```python
from build123d import *

# Parameters (mm, degrees)
SKETCH1_W           = 20
SKETCH1_H           = 20
SKETCH1_R           = 1.25
SKETCH1_R_2         = 2.625
BOSS_EXTRUDE1_DEPTH = 4


with BuildPart() as part:
    # Sketch1 → Boss-Extrude1 (new body)
    with BuildSketch(Plane(origin=(0, 0, 0), x_dir=(1, 0, 0), z_dir=(0, 1, 0))):
        with Locations((10, 10)):
            Rectangle(SKETCH1_W, SKETCH1_H)
        with Locations((17, 17)):
            Circle(SKETCH1_R, mode=Mode.SUBTRACT)
        with Locations((4.4625, 10)):
            Circle(SKETCH1_R_2, mode=Mode.SUBTRACT)
        with Locations((17, 3)):
            Circle(SKETCH1_R, mode=Mode.SUBTRACT)
        with BuildLine():
            Line((13.925, 7), (13.925, 13))
            ThreePointArc((13.925, 13), (15.5, 14.575), (17.075, 13))
            Line((17.075, 13), (17.075, 7))
            ThreePointArc((17.075, 7), (15.5, 5.425), (13.925, 7))
        make_face(mode=Mode.SUBTRACT)
        with BuildLine():
            Line((8.925, 7), (8.925, 13))
            ThreePointArc((8.925, 13), (10.5, 14.575), (12.075, 13))
            Line((12.075, 13), (12.075, 7))
            ThreePointArc((12.075, 7), (10.5, 5.425), (8.925, 7))
        make_face(mode=Mode.SUBTRACT)
    extrude(amount=-BOSS_EXTRUDE1_DEPTH)


solid = part.part
```
The listing builds one solid part. Answer for the finished solid, in the listing's coordinates (mm). A direction names the side the tool comes from. Give positions to 0.01 mm unless a question says otherwise; leave off trailing zeros. Order: outer loops, then holes, each group sorted by start corner. A loop starts at its lowest first (then second) coordinate and runs counter-clockwise, first axis right, second up.
1) Determine the mould class of faces 1 (the face through (10, -2, 0)), 2 (the face through (10.465, -1.972, -14.575)), 3 (the face through (8, -4, -10)) for opening direction Z: pulls with the +Z half, pulls with the -Z half, needs draft (parallel to the pull), parting line crosses it, or undercut.
Reported:
face 1: pulls with the +Z half
face 2: undercut
face 3: needs draft
2) Consider line 1 along X through (y, z) = (-0.3, -12.75) (3 decimals); line 2 along X through (y, z) = (-2.3, -10) (1 decimal); line 3 along Z through (x, y) = (4.5, -2). Determine where each line is inside the solid, lowest interval first.
Reported:
line 1: x = 0 to 8.925, 12.075 to 13.925, 17.075 to 20
line 2: x = 0 to 1.8, 7.1 to 8.9, 12.1 to 13.9, 17.1 to 20
line 3: z = -20 to -12.62, -7.38 to 0
3) Find section D-D on y = -3.15. Give the number of separate pieces and of enclosed holes in the cut face, then the cut area to 3 significant figures.
Reported:
separate pieces: 1
enclosed holes: 5
area: 315 mm2
4) Find section C-C on z = -17. Write down the section's boundary in (x, y), then the cut area to 3 significant figures.
Reported:
outline: (0, -4) - (15.75, -4) - (15.75, 0) - (0, 0) - close; (18.25, -4) - (20, -4) - (20, 0) - (18.25, 0) - close
area: 70.0 mm2
5) Find section B-B on x = 10.5. Write down the section's boundary in (y, z) (3 decimals), then the cut area to 3 significant figures.
Reported:
outline: (-4, -20) - (0, -20) - (0, -14.575) - (-4, -14.575) - close; (-4, -5.425) - (0, -5.425) - (0, 0) - (-4, 0) - close
area: 43.4 mm2
6) Given P1, Ø1.2, axis at y = -2.5, z = -11, coming from the -X side, flat-ended and moving along its own axis, determine where the tip first touches the part or whether it passes through.
Reported:
P1: stops at x = 0
7) Find section A-A on z = -10. Write down the section's boundary in (x, y) (1 decimal).
Reported:
outline: (0, -4) - (1.8, -4) - (1.8, 0) - (0, 0) - close; (7.1, -4) - (8.9, -4) - (8.9, 0) - (7.1, 0) - close; (12.1, -4) - (13.9, -4) - (13.9, 0) - (12.1, 0) - close; (17.1, -4) - (20, -4) - (20, 0) - (17.1, 0) - close
8) For faces 4 (the face through (20, -2, -10)), 5 (the face through (15.535, -1.972, -5.425)), determine the directions among +Z, -Z, +X, -X, +Y, -Y from which every point of the face is accessible in a straight line to the end or side of a thin tool.
Reported:
face 4: +Z, -Z, +X, +Y, -Y
face 5: +Y, -Y
